Model file for the job. Use its own axes, mm. A direction names the side the tool comes from. Round coordinates to 2 decimals unless told otherwise and drop trailing zeros. Loops run counter-clockwise (first coordinate to the right, second up) from the corner with the lowest first, then second, coordinate; pieces in that order, holes last. Notation, with made-up numbers: M -37.75,-20 L -10.75,-20 A18 ccw -10.75,-6 Z; hole C 32.5,-10.5 d6. An arc over 180 degrees is marked long. Use a Markdown table: item, result. Add a question column.
Item 1: Tool access for faces 1 (the flat face through (-17, 18.417, 1)), 2 (the flat face through (-15, 23.417, 1)): list every direction of +Z, -Z, +X, -X, +Y, -Y with a clear straight run to the whole face (end or side of a thin tool).
Item 2: Wall check: L1, parallel to Y at x = -8.25, z = 1.15; L2, parallel to Y at x = -8, z = 1.95; L3, parallel to X at y = 9, z = 0.5. Give the ranges that are in metal, low to high. Write a range as from..to.
Item 3: Saw through at D-D on z = 0.4. Write the cut outline in (x, y), then the cut area to 3 significant figures.
Item 4: Saw through at B-B on z = 1.65. Write the cut outline in (x, y), then the cut area to 3 significant figures.
Item 5: Two-plate mould, pull along X, no slides. Class faces 3 (the cylindrical face through (-8.585, 8.466, 1.521)), 4 (the cylindrical face through (-6.992, 19.677, 2.137)), 5 (the flat face through (-12, 19, 0)), 6 (the flat face through (-9.655, 11, 1)): +X half, -X half, draft (parallel to the pull), parting line (faces both ways), or undercut.
Item 6: Saw through at A-A on x = -18.25. Write the cut outline in (y, z).
Item 7: Saw through at C-C on y = 11.75. Write the cut outline in (x, z), then the cut area to 3 significant figures.
Item 8: Pin check, flat tips, straight feed: P1, Ø0.9, axis at y = 10.5, z = 1, coming from the -X side; P2, Ø2.5, axis at x = -19.15, y = 20.92, coming from the -Z side; P3, Ø3, axis at x = -7.15, y = 20.92, coming from the -Z side; P4, Ø1, axis at x = -10.5, z = 2.5, coming from the -Y side. Stop position of each tip, or through.
```python
from build123d import *

# Parameters (mm, degrees)
F1_DEPTH       = 3
F2_D           = 3
F3_D           = 2.5
F3_CSINK_D     = 5
F3_CSINK_ANGLE = 90


with BuildPart() as f1:
    # F0 (on Top) → F1 (new body)
    with BuildSketch(Plane.XY):
        Polygon((-4.6546061151, 23.416666063), (-24.6546061151, 23.416666063), (-24.6546061151, 18.416666063), (-9.6546061151, 18.416666063), align=None)
        Polygon((-4.6546061151, 3.416666063), (-4.6546061151, 23.416666063), (-9.6546061151, 18.416666063), (-9.6546061151, 3.416666063), align=None)
    extrude(amount=F1_DEPTH)

    # F2 (through all)
    with Locations(Plane(origin=(0, 0, 0), x_dir=(1, 0, 0), z_dir=(0, 0, -1))):
        with Locations((-7.1546061151, -8.916666063), (-19.1546061151, -20.916666063)):
            Hole(F2_D / 2)

    # F3 (through all)
    with Locations(Plane(origin=(0, 0, 0), x_dir=(1, 0, 0), z_dir=(0, 0, -1))):
        with Locations((-7.1546061151, -20.916666063)):
            CounterSinkHole(F3_D / 2, F3_CSINK_D / 2, counter_sink_angle=F3_CSINK_ANGLE)


solid = f1.part
```
Entries:
| question | item | result |
|---|---|---|
| 1 | face 1 | +Z, -Z, -X, -Y |
| 1 | face 2 | +Z, -Z, +X, -X, +Y |
| 2 | L1 | 3.42..7.89, 9.94..20.13, 21.71..23.42 |
| 2 | L2 | 3.42..7.68, 10.16..20, 21.84..23.42 |
| 2 | L3 | -9.65..-8.65, -5.66..-4.65 |
| 3 | outline | M -24.65,18.42 L -9.65,18.42 L -9.65,3.42 L -4.65,3.42 L -4.65,23.42 L -24.65,23.42 Z; hole C -19.15,20.92 d3; hole C -7.15,20.92 d4.2; hole C -7.15,8.92 d3 |
| 3 | area | 147 mm2 |
| 4 | outline | M -24.65,18.42 L -9.65,18.42 L -9.65,3.42 L -4.65,3.42 L -4.65,23.42 L -24.65,23.42 Z; hole C -19.15,20.92 d3; hole C -7.15,8.92 d3; hole C -7.15,20.92 d2.5 |
| 4 | area | 156 mm2 |
| 5 | face 3 | undercut |
| 5 | face 4 | undercut |
| 5 | face 5 | draft |
| 5 | face 6 | -X half |
| 6 | outline | M 18.42,0 L 19.72,0 L 19.72,3 L 18.42,3 Z; M 22.11,0 L 23.42,0 L 23.42,3 L 22.11,3 Z |
| 7 | outline | M -9.65,0 L -4.65,0 L -4.65,3 L -9.65,3 Z |
| 7 | area | 15.0 mm2 |
| 8 | P1 | x = -9.65 |
| 8 | P2 | through |
| 8 | P3 | z = 0.99 |
| 8 | P4 | y = 18.42 |
